Verification items for this drawing (mm, ordinates from the low corner). Coordinates: 2 decimals unless noted, no trailing zeros.
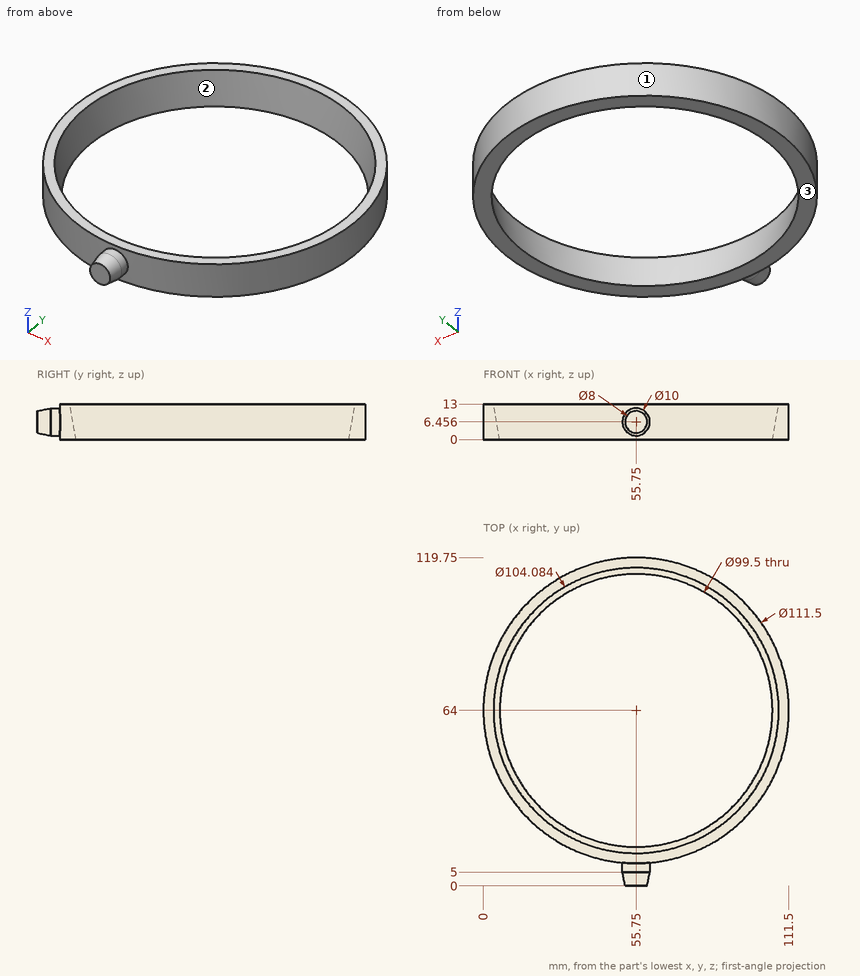
(1) Release check for a two-part mould opening along Y. For the marked faces 1, 2 and 3 record: +Y half, -Y half, draft (parallel to the pull), parting line (faces both ways), or undercut.
Filled in:
face 1: parting line
face 2: undercut
face 3: draft
(2) Thickness scan on probe 1 along Y at (x, z) = (55.75, 0.05); probe 2 along X at (y, z) = (6, 6.5); probe 3 along X at (y, z) = (107, 4.5) (1 decimal). Record the ranges inside material, lowest first.
Filled in:
probe 1: y = 8.25 to 14.24, 113.76 to 119.75
probe 2: x = 50.75 to 60.75
probe 3: x = 20.3 to 29.2, 82.3 to 91.2
(3) Go/stop test with flat-tipped pins: P1, Ø2, axis at y = 92.5, z = 5.5, coming from the -X side (1 decimal); P2, Ø6, axis at y = 21.5, z = 4.5, coming from the -X side; P3, Ø3, axis at x = 33.5, y = 17.5, coming from the +Z side; P4, Ø1.5, axis at x = 25, z = 10.5, coming from the +Y side. Record where each tip stops, or that it passes through.
Filled in:
P1: stops at x = 7.3
P2: stops at x = 16.41
P3: stops at z = 13
P4: stops at y = 110.99
